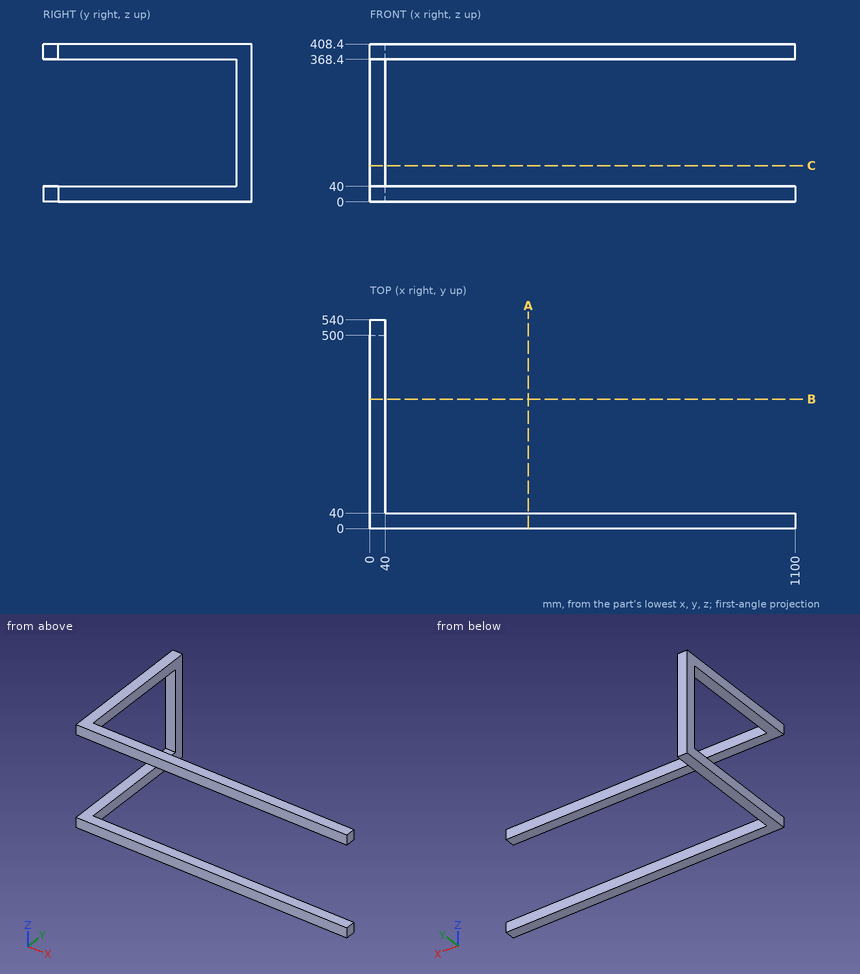
Job drawing, mm, ordinate dimensions from the low corner. One solid piece. Give positions to 0.01 mm unless a question says otherwise; leave off trailing zeros. Loops run counter-clockwise (first coordinate to the right, second up) from the corner with the lowest first, then second, coordinate; pieces in that order, holes last. Notation, with made-up numbers: M 42.5,-26 L 56.5,-26 A22 cw 56.5,-7 Z; hole C 44.5,18 d2. An arc over 180 degrees is marked long. Answer in a Markdown table with one row per item. Add a question column.
Item 1: Drop flat-ended pins along their axis: P1, Ø12, axis at x = 759, z = 17.5, coming from the +Y side; P2, Ø20, axis at x = 11.5, z = 143.5, coming from the -Y side; P3, Ø10, axis at y = 230.5, z = 359.5, coming from the -X side. Give the stop position or say it passes through.
Item 2: Band-saw the part on A-A on x = 410.5. Give the cut face in (y, z), then the cut area to 3 significant figures.
Item 3: Band-saw the part on C-C on z = 93.5. Give the cut face in (x, y), then the cut area to 3 significant figures.
Item 4: Probe probe 1 along Y at (x, z) = (566, 35). List the from-to ranges inside material, lowest first.
Reply:
| question | item | result |
|---|---|---|
| 1 | P1 | stops at y = 40 |
| 1 | P2 | stops at y = 500 |
| 1 | P3 | passes through |
| 2 | outline | M 0,0 L 40,0 L 40,40 L 0,40 Z; M 0,368.4 L 40,368.4 L 40,408.4 L 0,408.4 Z |
| 2 | area | 3,200 mm^2 |
| 3 | outline | M 0,500 L 40,500 L 40,540 L 0,540 Z |
| 3 | area | 1,600 mm^2 |
| 4 | probe 1 | y = 0 to 40 |
